Autodesk Inventor part; units mm, degrees
ref_plane "YZ Plane" through (0, 0, 0) normal (1, 0, 0) x (0, 1, 0)
ref_plane "XZ Plane" through (0, 0, 0) normal (0, 1, 0) x (-1, 0, 0)
ref_plane "XY Plane" through (0, 0, 0) normal (0, 0, 1) x (1, 0, 0)
ref_plane "Work Plane1" through (0, 0, -12) normal (0, 0, 1) x (1, 0, 0)
ref_plane "Work Plane2" through (101.5856, 16.1884, -33.1044) normal (0, 0, 1) x (1, 0, 0)
sketch "Sketch2" plane through (101.5856, 16.1884, -33.1044) normal (0, 0, 1) x (1, 0, 0)
  line L0 (30.5, -15.5) -> (30.5, 15.5)
  arc A0 (30.5, 15.5) -> (29.5, 16.5) centre (29.5, 15.5) ccw
  line L1 (29.5, 16.5) -> (-29.5, 16.5)
  arc A1 (-29.5, 16.5) -> (-30.5, 15.5) centre (-29.5, 15.5) ccw
  line L2 (-30.5, 15.5) -> (-30.5, -15.5)
  arc A2 (-30.5, -15.5) -> (-29.5, -16.5) centre (-29.5, -15.5) ccw
  line L3 (-29.5, -16.5) -> (29.5, -16.5)
  arc A3 (29.5, -16.5) -> (30.5, -15.5) centre (29.5, -15.5) ccw
  line L4 (-28, 13) -> (-28, -13)
  arc A4 (-27, 14) -> (-28, 13) centre (-27, 13) ccw
  line L5 (27, 14) -> (-27, 14)
  arc A5 (28, 13) -> (27, 14) centre (27, 13) ccw
  line L6 (28, -13) -> (28, 13)
  arc A6 (27, -14) -> (28, -13) centre (27, -13) ccw
  line L7 (-27, -14) -> (27, -14)
  arc A7 (-28, -13) -> (-27, -14) centre (-27, -13) ccw
  line L8 (-29.3, 5.25) -> (-29.3, -5.25)
  line L9 (-29.3, -5.25) -> (-28, -5.25)
  line L10 (-28, 5.25) -> (-28, -5.25)
  line L11 (-29.3, 5.25) -> (-28, 5.25)
  line L12 (28, 5.25) -> (28, -5.25)
  line L13 (28, -5.25) -> (29.3, -5.25)
  line L14 (29.3, 5.25) -> (29.3, -5.25)
  line L15 (28, 5.25) -> (29.3, 5.25)
  point P0 (-101.5856, -16.1884)
extrude "Extrusion2" add sketch "Sketch2" along normal blind 5
chamfer "Chamfer2" distance 1 angle 45 16 edges at (101.5856, 30.1884, -33.1044) (129.2927, 29.8955, -33.1044) (129.5856, 25.3134, -33.1044) (73.8785, 29.8955, -33.1044) (73.5856, 25.3134, -33.1044) (101.5856, 2.1884, -33.1044) (73.8785, 2.4813, -33.1044) (73.5856, 7.0634, -33.1044) (129.2927, 2.4813, -33.1044) (129.5856, 7.0634, -33.1044) (130.2356, 21.4384, -33.1044) (130.2356, 10.9384, -33.1044) (130.8856, 16.1884, -33.1044) (72.9356, 21.4384, -33.1044) (72.2856, 16.1884, -33.1044) (72.9356, 10.9384, -33.1044)
properties part number "ledy_bateryjki_ramka_check"
Source: CAD feature listing. Evaluate the final solid. Frame: model axes, mm. A direction names the side the tool comes from. Give positions to 0.01 mm unless a question says otherwise; leave off trailing zeros. Loops run counter-clockwise (first coordinate to the right, second up) from the corner with the lowest first, then second, coordinate; pieces in that order, holes last. Notation, with made-up numbers: (-25, -30) - (-5, -30) arc R26 ccw to (-5, 8) - close; hole circle Ø2 at (-33.5, 37). An arc over 180 degrees is marked (long way). Use CSV: the item, a comma, the result in double quotes. Start each with the question number.
1. Reachability of faces 4 (the flat face through (71.086, 16, -31)), 5 (the conical face through (129.58, 2.21, -32.5)), 6 (the flat face through (130.886, 16, -30)) from +Z, -Z, +X, -X, +Y, -Y: full face, straight path, thin tool, end or side. Return the list, or none.
2. Section C-C (z = -30.3). Output: boundary loops of the cut face in (x, y).
3. Section A-A (x = 88). Output: boundary loops of the cut face in (y, z).
4. Ray query, L1, parallel to Y at x = 120, z = -31.4; L2, parallel to X at y = 13.5, z = -28.6; L3, parallel to X at y = 25, z = -31.3. Return the intervals inside material, ascending.
5. Section B-B (y = 18.5). Output: boundary loops of the cut face in (x, z), then the cut area to 3 significant figures.
6. Draft query along Y for faces 1 (the conical face through (73.6, 2.2, -32.5)), 2 (the flat face through (101, -0.312, -31)), 3 (the flat face through (132.086, 16, -31)). Return one class per face: +Y half, -Y half, draft (parallel to the pull), parting line (faces both ways), or undercut.
Response:
1,face 4,"+Z, -Z, -X, +Y, -Y"
1,face 5,"-Z"
1,face 6,"+Z, -Z"
2,outline,"(71.09, 0.69) arc R1 ccw to (72.09, -0.31) - (131.09, -0.31) arc R1 ccw to (132.09, 0.69) - (132.09, 31.69) arc R1 ccw to (131.09, 32.69) - (72.09, 32.69) arc R1 ccw to (71.09, 31.69) - close; hole (72.29, 10.94) - (73.59, 10.94) - (73.59, 3.19) arc R1 ccw to (74.59, 2.19) - (128.59, 2.19) arc R1 ccw to (129.59, 3.19) - (129.59, 10.94) - (130.89, 10.94) - (130.89, 21.44) - (129.59, 21.44) - (129.59, 29.19) arc R1 ccw to (128.59, 30.19) - (74.59, 30.19) arc R1 ccw to (73.59, 29.19) - (73.59, 21.44) - (72.29, 21.44) - close"
3,outline,"(-0.31, -33.1) - (1.19, -33.1) - (2.19, -32.1) - (2.19, -28.1) - (-0.31, -28.1) - close; (30.19, -32.1) - (31.19, -33.1) - (32.69, -33.1) - (32.69, -28.1) - (30.19, -28.1) - close"
4,L1,"-0.31 to 2.19, 30.19 to 32.69"
4,L2,"71.09 to 72.29, 130.89 to 132.09"
4,L3,"71.09 to 73.59, 129.59 to 132.09"
5,outline,"(71.09, -33.1) - (71.29, -33.1) - (72.29, -32.1) - (72.29, -28.1) - (71.09, -28.1) - close; (130.89, -32.1) - (131.89, -33.1) - (132.09, -33.1) - (132.09, -28.1) - (130.89, -28.1) - close"
5,area,"11.0 mm²"
6,face 1,"undercut"
6,face 2,"-Y half"
6,face 3,"draft"
